Can you work these out from the model? Positions are in its coordinate system, mm. Face numbers are marked on the shaded views. A direction names the side the tool comes from. Coordinates: 2 decimals unless noted, no trailing zeros. Order: outer loops, then holes, each group sorted by start corner. A loop starts at its lowest first (then second) coordinate and runs counter-clockwise, first axis right, second up. Notation, with made-up numbers: (51, 26) -> (87, 26) arc R16 ccw to (87, 49) -> close; hole circle Ø4 at (-22, 71). An arc over 180 degrees is marked (long way). Return JSON: item names as keys, results as strings. Group by question number.
1) If we section it at B-B, the plane x = 0: Please give me the cut outline in (y, z) (3 decimals), then the cut area to 3 significant figures.
2) If I drill on probe 1 along Z at (x, y) = (-0.5, 0) (3 decimals); probe 2 along Z at (x, y) = (2, 3) (3 decimals); probe 3 along X at (y, z) = (-1, -2), over which ranges is the centre line in solid material (lowest first)? Write a range as from..to.
3) For the marked faces 1 and 2, which set-ups out of +Z, -Z, +X, -X, +Y, -Y let a thin tool reach every point of the face, with its end or its side?
4) For pin 1 (2 mm diameter, centred on x = -3.5, z = -9.5, fed in from +Y); pin 2 (1.5 mm diameter, centred on y = -3.5, z = -7, fed in from +X), each with a flat end and sliding along its axis, tell me the tip position at first contact or that it passes through.
5) If we section it at C-C, the plane z = -13.25: Please give me the cut outline in (x, y) (3 decimals).
6) If we section it at A-A, the plane y = 0: Please give me the cut outline in (x, z) (3 decimals).
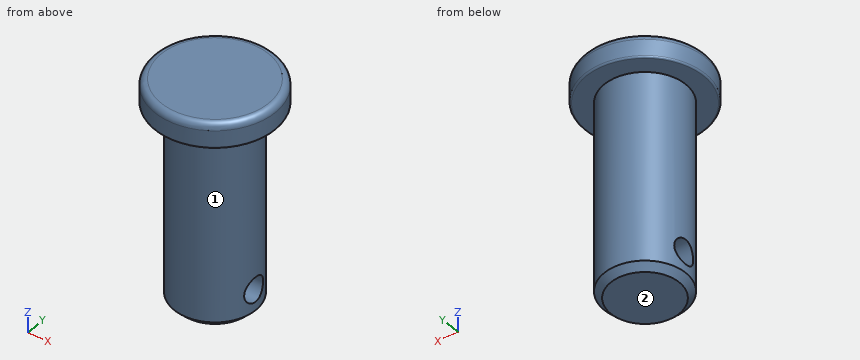
from build123d import *

# Parameters (mm, degrees)
SKETCH2_R           = 0.9652
EXTRUDE1_DEPTH      = 5.699
EXTRUDE1_DEPTH_BACK = 5.6990001


with BuildPart() as part:
    # Sketch1 → Revolve Base (revolve)
    with BuildSketch(Plane(origin=(0, 0, 0), x_dir=(0, 0, -1), z_dir=(1, 0, 0))):
        with BuildLine():
            Line((0, 0), (0, 4.191))
            ThreePointArc((0, 4.191), (0.148789755, 4.550210245), (0.508, 4.699))
            Line((0.508, 4.699), (1.778, 4.699))
            ThreePointArc((1.778, 4.699), (1.867802561, 4.661802561), (1.905, 4.572))
            Line((1.905, 4.572), (1.905, 3.175))
            Line((1.905, 3.175), (16.637, 3.175))
            Line((16.637, 3.175), (17.145, 2.667))
            Line((17.145, 2.667), (17.145, 0))
            Line((17.145, 0), (0, 0))
        make_face()
    revolve(axis=Axis((0, 0, 0), (0, 0, -1)))

    # Sketch2 → Extrude1 (cut, two sides)
    with BuildSketch(Plane(origin=(0, 0, 0), x_dir=(0, 0, -1), z_dir=(1, 0, 0))) as extrude1_sk:
        with Locations((15.0114, 0)):
            Circle(SKETCH2_R)
    extrude(amount=EXTRUDE1_DEPTH, mode=Mode.SUBTRACT)
    extrude(extrude1_sk.sketch, amount=-EXTRUDE1_DEPTH_BACK, mode=Mode.SUBTRACT)


solid = part.part
Result sheet:
{
 "1": {"outline": "(-4.699, -1.778) arc R0.127 ccw to (-4.572, -1.905) -> (-3.175, -1.905) -> (-3.175, -16.637) -> (-2.667, -17.145) -> (2.667, -17.145) -> (3.175, -16.637) -> (3.175, -1.905) -> (4.572, -1.905) arc R0.127 ccw to (4.699, -1.778) -> (4.699, -0.508) arc R0.508 ccw to (4.191, 0) -> (-4.191, 0) arc R0.508 ccw to (-4.699, -0.508) -> close; hole circle Ø1.93 at (0, -15.011)", "area": "111 mm2"},
 "2": {"probe 1": "z = -17.145..-15.977, -14.046..0", "probe 2": "z = -1.905..0", "probe 3": "x = -3.01..3.01"},
 "3": {"face 1": "-Z", "face 2": "-Z, +X, -X, +Y, -Y"},
 "4": {"pin 1": "stops at y = 1.96", "pin 2": "stops at x = 1.59"},
 "5": {"outline": "circle Ø6.35 at (0, 0)"},
 "6": {"outline": "(-4.699, -1.778) arc R0.127 ccw to (-4.572, -1.905) -> (-3.175, -1.905) -> (-3.175, -14.046) -> (3.175, -14.046) -> (3.175, -1.905) -> (4.572, -1.905) arc R0.127 ccw to (4.699, -1.778) -> (4.699, -0.508) arc R0.508 ccw to (4.191, 0) -> (-4.191, 0) arc R0.508 ccw to (-4.699, -0.508) -> close; (-3.175, -16.637) -> (-2.667, -17.145) -> (2.667, -17.145) -> (3.175, -16.637) -> (3.175, -15.977) -> (-3.175, -15.977) -> close"}
}
